Part model, mm, in its own coordinate system. Round coordinates to 2 decimals unless told otherwise and drop trailing zeros. Order: outer loops, then holes, each group sorted by start corner. A loop starts at its lowest first (then second) coordinate and runs counter-clockwise, first axis right, second up. Notation, with made-up numbers: (-24.5, 39) - (-5.5, 39) arc R19 ccw to (-5.5, 59) - close; hole circle Ø9 at (54.5, 44). An arc over 180 degrees is marked (long way). Answer as a JSON object with one key per item and string values.
Solid Edge part; units mm, degrees
sketch "Sketch1" plane through (0, 0, 0) normal (1, 0, 0) x (0, 1, 0)
  line L0 (-70.6829, -217.8929) -> (-40.6829, -217.8929)
  line L1 (-40.6829, -217.8929) -> (-40.6829, 12.1071)
  line L2 (-40.6829, 12.1071) -> (-70.6829, 12.1071)
  line L3 (-70.6829, 12.1071) -> (-70.6829, -217.8929)
  line L4 (-70.6829, 12.1071) -> (-40.6829, 12.1071)
  line L5 (-54.1753, 28.1984) -> (-40.6829, 12.1071)
  line L6 (-57.1901, 28.1988) -> (-54.1753, 28.1984)
  line L7 (-70.6829, 12.1071) -> (-57.1901, 28.1988)
  dimension "D1" = 70.6829
  dimension "D2" = 54.1753
  dimension "D3" = 70.6829
  dimension "D4" = 40.6829
  dimension "D5" = 40.6829
  dimension "D6" = 0
extrude "Protrusion1" add sketch "Sketch1" against normal blind 3
sketch "Sketch2" plane through (0, -21.8205, 20.1807) normal (1, 0, 0) x (0, 1, 0)
  circle A0 centre (-33.8622, -156.9821) radius 5
  circle A1 centre (-33.8621, -1.9821) radius 5
extrude "ExtrudedProtrusion_2" add sketch "Sketch2" along normal blind 11
mirror "Mirror1" about plane through (5, -21.8205, 20.1506) normal (1, 0, 0) of "Protrusion1"
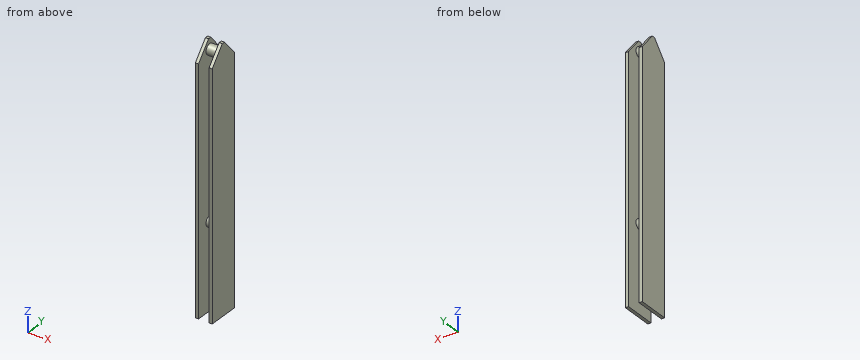
Item 1: Cut at A-A (z = -146). Write the cut outline in (x, y), plus the area to 3 significant figures.
Taken from the geometry:
{"outline": "(-3, -70.68) - (0, -70.68) - (0, -40.68) - (-3, -40.68) - close; (10, -70.68) - (13, -70.68) - (13, -40.68) - (10, -40.68) - close", "area": "180 mm2"}
Item 2: Cut at C-C (x = 3). Write the cut outline in (y, z).
Taken from the geometry:
{"outline": "circle Ø10 at (-55.68, -136.8); circle Ø10 at (-55.68, 18.2)"}
Item 3: Drop a flat-ended pin along its axis: P1, Ø3, axis at x = -1, y = -45.5, coming from the +Z side. Give the stop position or say it passes through.
Taken from the geometry:
{"P1": "z = 19.64"}
Item 4: Probe L1, parallel to X at y = -49, z = -97; L2, parallel to Z at x = 1.25, y = -53.5; L3, parallel to Z at x = 11.5, y = -68. List the from-to ranges inside material, lowest first. Write a range as from..to.
Taken from the geometry:
{"L1": "-3..0, 10..13", "L2": "-141.3..-132.3, 13.7..22.7", "L3": "-217.89..15.31"}
Item 5: Cut at B-B (y = -47.5). Write the cut outline in (x, z), plus the area to 3 significant figures.
Taken from the geometry:
{"outline": "(-3, -217.89) - (0, -217.89) - (0, 20.24) - (-3, 20.24) - close; (10, -217.89) - (13, -217.89) - (13, 20.24) - (10, 20.24) - close", "area": "1,430 mm2"}
